Geometry check sheet. Reference: the model listing, model coordinates, mm. Round coordinates to 2 decimals unless told otherwise and drop trailing zeros. Loops run counter-clockwise (first coordinate to the right, second up) from the corner with the lowest first, then second, coordinate; pieces in that order, holes last. Notation, with made-up numbers: M 49,42 L 75,42 A22 cw 75,51 Z; hole C 80.5,85.25 d5. An arc over 180 degrees is marked long. Use one line per item in the form item = value. Start each with the question number.
1. Material ranges on line 1 (X direction, y = 8.5, z = -13.5); line 2 (Y direction, x = 40, z = 0); line 3 (Z direction, x = 131.5, y = -13), recorded low to high.
2. Cross-section at A-A (z = 0). Record the boundary of the cut face in (x, y), then the cut area to 3 significant figures.
3. Go/stop test with flat-tipped pins: pin 1 (5 mm diameter, centred on x = 21, z = 8.5, fed in from +Y); pin 2 (1.5 mm diameter, centred on x = 18.5, y = 10, fed in from +Z); pin 3 (1 mm diameter, centred on x = -66.5, z = 1, fed in from +Y). Record where each tip stops, or that it passes through.
4. Cross-section at C-C (x = 79). Record the boundary of the cut face in (y, z).
5. Cross-section at D-D (y = -14.5). Record the boundary of the cut face in (x, z).
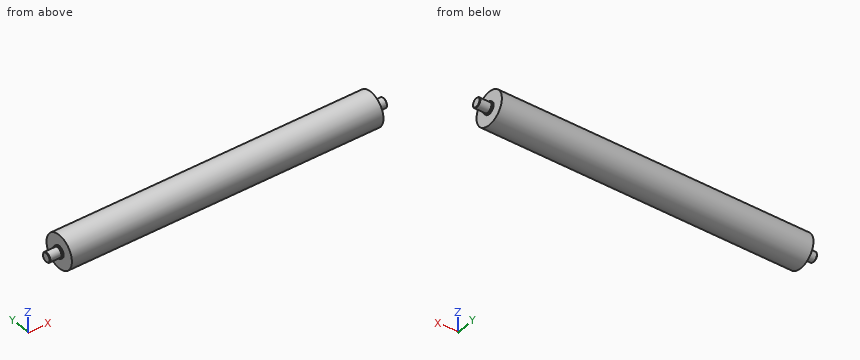
```python
from build123d import *

# Parameters (mm, degrees)
CHAMFER_1_SIZE = 0.5


with BuildPart() as part:
    # 草图1 → 旋转1 (revolve)
    with BuildSketch(Plane(origin=(0, 0, 0), x_dir=(1, 0, 0), z_dir=(0, 1, 0)), mode=Mode.PRIVATE) as revolve_1_sk:
        Polygon((-176, 0), (176, 0), (176, 5), (164, 5), (164, 6.15), (162.5, 6.15), (162.5, 17.5), (-162.5, 17.5), (-162.5, 6.15), (-164, 6.15), (-164, 5), (-176, 5), align=None)
    revolve(revolve_1_sk.sketch.rotate(Axis((-176, 0, 0), (1, 0, 0)), 180), axis=Axis((-176, 0, 0), (1, 0, 0)))

    # 倒角1
    chamfer_1_edges = [part.edges().sort_by_distance(p)[0] for p in [
        (176, 0, -5),
        (-176, 0, -5),
    ]]
    chamfer(chamfer_1_edges, length=CHAMFER_1_SIZE)


solid = part.part
```
Reported:
q1.line_1 = -162.5 to 162.5
q1.line_2 = -17.5 to 17.5
q1.line_3 = -11.72 to 11.72
q2.outline = M -176,-4.5 L -175.5,-5 L -164,-5 L -164,-6.15 L -162.5,-6.15 L -162.5,-17.5 L 162.5,-17.5 L 162.5,-6.15 L 164,-6.15 L 164,-5 L 175.5,-5 L 176,-4.5 L 176,4.5 L 175.5,5 L 164,5 L 164,6.15 L 162.5,6.15 L 162.5,17.5 L -162.5,17.5 L -162.5,6.15 L -164,6.15 L -164,5 L -175.5,5 L -176,4.5 Z
q2.area = 11,700 mm²
q3.pin_1 = 16.44
q3.pin_2 = 14.86
q3.pin_3 = 17.49
q4.outline = C 0,0 d35
q5.outline = M -162.5,-9.8 L 162.5,-9.8 L 162.5,9.8 L -162.5,9.8 Z
